Model file for the job. Use its own axes, mm. A direction names the side the tool comes from. Coordinates: 2 decimals unless noted, no trailing zeros.
from build123d import *

# Parameters (mm, degrees)
SKETCH1_W           = 101.6
SKETCH1_H           = 101.6
BOSS_EXTRUDE1_DEPTH = 76.2
SKETCH2_R           = 6.477
SKETCH2_R_2         = 1.27
CUT_EXTRUDE1_DEPTH  = 12.7


with BuildPart() as part:
    # Sketch1 → Boss-Extrude1 (new, symmetric)
    with BuildSketch(Plane(origin=(0, 0, 0), x_dir=(1, 0, 0), z_dir=(0, 1, 0))):
        Rectangle(SKETCH1_W, SKETCH1_H)
    extrude(amount=BOSS_EXTRUDE1_DEPTH, both=True)

    # Sketch2 → Cut-Extrude1 (cut)
    with BuildSketch(Plane(origin=(0, 76.2, 0), x_dir=(1, 0, 0), z_dir=(0, 1, 0))):
        with Locations(Location((0, 0, 0), (0, 0, 270))):
            Circle(SKETCH2_R)
        with Locations(Location((0, 10.3251, 0), (0, 0, 270))):
            Circle(SKETCH2_R_2)
        with Locations(Location((0, -10.3251, 0), (0, 0, 270))):
            Circle(SKETCH2_R_2)
    extrude(amount=-CUT_EXTRUDE1_DEPTH, mode=Mode.SUBTRACT)


solid = part.part
Q1. Drill centre line: line 1 (X direction, y = 67.25, z = 0). Where is it in solid material? Low to high.
Answers:
line 1: x = -50.8 to -6.48, 6.48 to 50.8
Q2. Mould opens along Z. For faces 3 (the cylindrical face through (-6.323, 69.939, -1.404)), 4 (the flat face through (-50.8, 1, 1)), 5 (the flat face through (-1, 1, 50.8)) say: +Z half, -Z half, draft (parallel to the pull), parting line (faces both ways), or undercut.
Answers:
face 3: undercut
face 4: draft
face 5: +Z half
Q3. Flat gauge pin, fed straight in: P1, Ø0.8, axis at x = 0.5, z = -9.5, coming from the +Y side. Where does the tip first touch, or does it go through?
Answers:
P1: stops at y = 76.2
Q4. Which spindle directions (+Z, -Z, +X, -X, +Y, -Y) get a long thin tool onto all of the face, cutting with end or side? Do faces 1 (the flat face through (0, 63.5, 0)), 2 (the flat face through (-1, -76.2, -1)). Say none if no direction does.
Answers:
face 1: +Y
face 2: +Z, -Z, +X, -X, -Y
